Here's how the part is built. I have some questions about the finished solid (model axes, mm). Face numbers are marked on the shaded views. A direction names the side the tool comes from. Coordinates: 2 decimals unless noted, no trailing zeros. Write each loop counter-clockwise with the first axis right and the second up, starting at its lowest first coordinate (ties: lowest second). Pieces come first, ordered by that corner, then holes.
(1) Please list where these lines run through material, in increasing order: probe 1 along Y at (x, z) = (36, 48); probe 2 along X at (y, z) = (23, 12); probe 3 along Z at (x, y) = (24, 10).
(2) Imagine slicing it at A-A, the plane z = 24.5. List the corners of the cut face in (x, y) for me.
(3) Thinking about a two-plate mould opening in Z: for the marked faces 1, 2 and 3, which applies, released by +Z, released by -Z, zero draft, split by the parting line, or undercut?
(4) Imagine slicing it at D-D, the plane z = 30.5. List the corners of the cut face in (x, y) for me.
(5) Which directions (+Z, -Z, +X, -X, +Y, -Y) give clear straight access to the entire face, cutting with the end or side of a thin tool? Please do the marked faces 4, 5 and 6.
(6) Imagine slicing it at B-B, the plane x = 18. List the corners of the cut face in (y, z) for me.
(7) Imagine slicing it at C-C, the plane y = 8.5. List the corners of the cut face in (x, z) for me, plus the area to 3 significant figures.
(8) For pin 1 Ø1 at (x, y) = (9, 15) entering from +Z; pin 2 Ø7.5 at (x, y) = (-6.5, 8.5) entering from -Z; pin 3 Ø4 at (y, z) = (18, 3.5) entering from +X, each with a flat end and sliding along its axis, tell me the tip position at first contact or that it passes through.
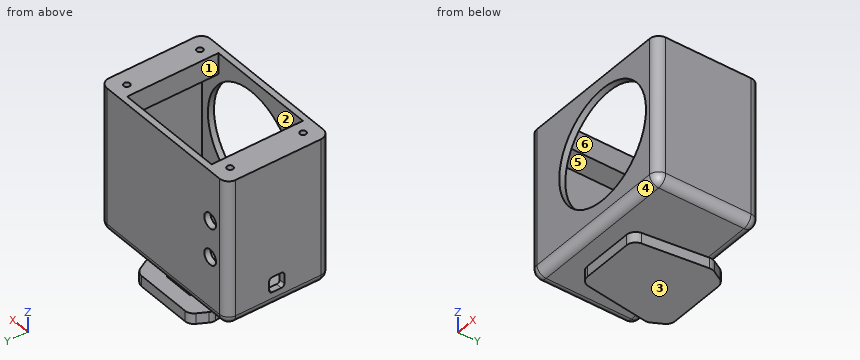
```python
from build123d import *

# Parameters (mm, degrees)
BOSS_EXTRUDE1_DEPTH  = 3.5
SKETCH2_W            = 10
SKETCH2_H            = 3
BOSS_EXTRUDE2_DEPTH  = 5
SKETCH3_W            = 50
SKETCH3_H            = 24
BOSS_EXTRUDE3_DEPTH  = 3
SKETCH4_W            = 50
SKETCH4_H            = 3
BOSS_EXTRUDE4_DEPTH  = 35
SKETCH5_W            = 4
SKETCH5_H            = 29
CUT_EXTRUDE3_DEPTH   = 35
FILLET1_R            = 2
SKETCH6_R            = 3.175
BOSS_EXTRUDE6_DEPTH  = 35
FILLET2_R            = 3
SKETCH8_W            = 10
SKETCH8_H            = 5
BOSS_EXTRUDE7_DEPTH  = 10
SKETCH9_W            = 10
SKETCH9_H            = 5
BOSS_EXTRUDE8_DEPTH  = 10
SKETCH10_W           = 53.514300768
SKETCH10_H           = 42.489179877
CUT_EXTRUDE4_DEPTH   = 20
BOSS_EXTRUDE9_DEPTH  = 40
SKETCH13_W           = 40
SKETCH13_H           = 10
BOSS_EXTRUDE10_DEPTH = 20
SKETCH14_W           = 4
SKETCH14_H           = 20
CUT_EXTRUDE7_DEPTH   = 20
FILLET3_R            = 2
SKETCH16_W           = 40
SKETCH16_H           = 10
CUT_EXTRUDE9_DEPTH   = 4
SKETCH19_W           = 40
SKETCH19_H           = 10
CUT_EXTRUDE10_DEPTH  = 24
SKETCH20_W           = 4
SKETCH20_H           = 2
CUT_EXTRUDE11_DEPTH  = 44
FILLET4_R            = 10
SKETCH21_W           = 58
SKETCH21_H           = 24
BOSS_EXTRUDE11_DEPTH = 2
SKETCH22_W           = 54.310686521
SKETCH22_H           = 40
CUT_EXTRUDE14_DEPTH  = 57
SKETCH24_W           = 10
SKETCH24_H           = 5
CUT_EXTRUDE15_DEPTH  = 5
SKETCH25_W           = 52
SKETCH25_H           = 2
BOSS_EXTRUDE12_DEPTH = 45
SKETCH26_W           = 2
SKETCH26_H           = 45
BOSS_EXTRUDE13_DEPTH = 22
SKETCH27_R           = 2.5
CUT_EXTRUDE16_DEPTH  = 45
SKETCH29_W           = 2
SKETCH29_H           = 45
BOSS_EXTRUDE14_DEPTH = 10
SKETCH30_W           = 45
SKETCH30_H           = 2
BOSS_EXTRUDE15_DEPTH = 50
SKETCH31_R           = 18.5
CUT_EXTRUDE17_DEPTH  = 60
SKETCH32_W           = 3
SKETCH32_H           = 34
BOSS_EXTRUDE17_DEPTH = 2
SKETCH33_W           = 2
SKETCH33_H           = 34
BOSS_EXTRUDE18_DEPTH = 45
BOSS_EXTRUDE20_REACH = 76.256
SKETCH37_W           = 7
SKETCH37_H           = 7
SKETCH38_R           = 1
CUT_EXTRUDE18_DEPTH  = 16
FILLET5_R            = 3
FILLET6_R            = 3
SKETCH39_W           = 5
SKETCH39_H           = 5
CUT_EXTRUDE22_DEPTH  = 10
FILLET7_R            = 1
SKETCH40_W           = 7
SKETCH40_H           = 30
BOSS_EXTRUDE21_DEPTH = 0.2


# Some blends are built 0.0001 mm under size
with BuildPart() as part:
    # Sketch1 → Boss-Extrude1 (new body)
    with BuildSketch(Plane.XY):
        Polygon((0, 24), (3, 0), (25, 0), (28, 24), (25, 29.5), (3, 29.5), align=None)
    extrude(amount=-BOSS_EXTRUDE1_DEPTH)

    # Sketch2 → Boss-Extrude2 (add)
    with BuildSketch(Plane.XY):
        with Locations((14, 18)):
            Rectangle(SKETCH2_W, SKETCH2_H)
    extrude(amount=BOSS_EXTRUDE2_DEPTH)

    # Sketch3 → Boss-Extrude3 (add)
    with BuildSketch(Plane.XY.offset(5)):
        with Locations((14, 17.5)):
            Rectangle(SKETCH3_W, SKETCH3_H)
    extrude(amount=BOSS_EXTRUDE3_DEPTH)

    # Sketch4 → Boss-Extrude4 (add)
    with BuildSketch(Plane.XY.offset(8)):
        with Locations((14, 28)):
            Rectangle(SKETCH4_W, SKETCH4_H)
    extrude(amount=BOSS_EXTRUDE4_DEPTH)

    # Sketch5 → Cut-Extrude3 (cut)
    with BuildSketch(Plane(origin=(0, 29.5, 0), x_dir=(1, 0, 0), z_dir=(0, 1, 0))):
        with Locations((-6, -25.5)):
            Rectangle(SKETCH5_W, SKETCH5_H)
    extrude(amount=-CUT_EXTRUDE3_DEPTH, mode=Mode.SUBTRACT)

    # Fillet1
    fillet1_edges = [part.edges().sort_by_distance(p)[0] for p in [
        (-8, 28, 40),
        (-4, 28, 40),
        (-4, 28, 11),
        (-8, 28, 11),
    ]]
    fillet(fillet1_edges, radius=FILLET1_R - 0.0001)  # a hair under: the kernel refuses the full size

    # Sketch6 → Boss-Extrude6 (add)
    with BuildSketch(Plane(origin=(39, 0, 0), x_dir=(0, 0, -1), z_dir=(1, 0, 0))):
        with BuildLine():
            Line((-29.274917218, 38.5), (-43, 29.5))
            Line((-43, 29.5), (-5, 29.5))
            Line((-5, 29.5), (-21.725082782, 38.5))
            ThreePointArc((-21.725082782, 38.5), (-25.5, 40), (-29.274917218, 38.5))
        make_face()
        with Locations((-25.5, 34.5)):
            Circle(SKETCH6_R, mode=Mode.SUBTRACT)
    extrude(amount=-BOSS_EXTRUDE6_DEPTH)

    # Fillet2
    fillet2_edges = [part.edges().sort_by_distance(p)[0] for p in [
        (25, 0, -1.75),
        (3, 0, -1.75),
        (0, 24, -1.75),
        (3, 29.5, -1.75),
        (25, 29.5, -1.75),
        (28, 24, -1.75),
    ]]
    fillet(fillet2_edges, radius=FILLET2_R)

    # Sketch8 → Boss-Extrude7 (add)
    with BuildSketch(Plane(origin=(0, 19.5, 0), x_dir=(1, 0, 0), z_dir=(0, 1, 0))):
        with Locations((14, -2.5)):
            Rectangle(SKETCH8_W, SKETCH8_H)
    extrude(amount=BOSS_EXTRUDE7_DEPTH)

    # Sketch9 → Boss-Extrude8 (add)
    with BuildSketch(Plane.XZ.offset(-16.5)):
        with Locations((14, 2.5)):
            Rectangle(SKETCH9_W, SKETCH9_H)
    extrude(amount=BOSS_EXTRUDE8_DEPTH)

    # Sketch10 → Cut-Extrude4 (cut)
    with BuildSketch(Plane(origin=(0, 29.5, 0), x_dir=(1, 0, 0), z_dir=(0, 1, 0))):
        with Locations((30.757150384, -26.244589939)):
            Rectangle(SKETCH10_W, SKETCH10_H)
    extrude(amount=CUT_EXTRUDE4_DEPTH, mode=Mode.SUBTRACT)

    # Sketch11 → Boss-Extrude9 (add)
    with BuildSketch(Plane(origin=(39, 0, 0), x_dir=(0, 0, -1), z_dir=(1, 0, 0))):
        with BuildLine():
            Line((-43, 39.5), (-43, 29.5))
            Line((-43, 29.5), (-24, 29.5))
            Line((-24, 29.5), (-24, 34.5))
            ThreePointArc((-24, 34.5), (-27.535533906, 35.964466094), (-29, 39.5))
            Line((-29, 39.5), (-43, 39.5))
        make_face()
        with BuildLine():
            Line((-24, 34.5), (-24, 29.5))
            Line((-24, 29.5), (-5, 29.5))
            Line((-5, 29.5), (-5, 39.5))
            Line((-5, 39.5), (-19, 39.5))
            ThreePointArc((-19, 39.5), (-20.464466094, 35.964466094), (-24, 34.5))
        make_face()
    extrude(amount=-BOSS_EXTRUDE9_DEPTH)

    # Sketch13 → Boss-Extrude10 (add)
    with BuildSketch(Plane.XY.offset(43)):
        with Locations((19, 34.5)):
            Rectangle(SKETCH13_W, SKETCH13_H)
        Polygon((-1, 29.5), (-11, 29.5), (-11, 26.5), (39, 26.5), (39, 29.5), align=None)
    extrude(amount=BOSS_EXTRUDE10_DEPTH)

    # Sketch14 → Cut-Extrude7 (cut)
    with BuildSketch(Plane(origin=(0, 29.5, 0), x_dir=(1, 0, 0), z_dir=(0, 1, 0))):
        with Locations((-6, -48)):
            Rectangle(SKETCH14_W, SKETCH14_H)
    extrude(amount=-CUT_EXTRUDE7_DEPTH, mode=Mode.SUBTRACT)

    # Fillet3
    fillet3_edges = [part.edges().sort_by_distance(p)[0] for p in [
        (-8, 28, 58),
        (-4, 28, 58),
    ]]
    fillet(fillet3_edges, radius=FILLET3_R - 0.0001)  # a hair under: the kernel refuses the full size

    # Sketch16 → Cut-Extrude9 (cut)
    with BuildSketch(Plane(origin=(0, 0, 5), x_dir=(-1, 0, 0), z_dir=(0, 0, -1))):
        with Locations((-19, 34.5)):
            Rectangle(SKETCH16_W, SKETCH16_H)
    extrude(amount=-CUT_EXTRUDE9_DEPTH, mode=Mode.SUBTRACT)

    # Sketch19 → Cut-Extrude10 (cut)
    with BuildSketch(Plane.XY.offset(63)):
        with Locations((19, 34.5)):
            Rectangle(SKETCH19_W, SKETCH19_H)
    extrude(amount=-CUT_EXTRUDE10_DEPTH, mode=Mode.SUBTRACT)

    # Sketch20 → Cut-Extrude11 (cut)
    with BuildSketch(Plane.XY.offset(39)):
        with Locations((6, 31.5)):
            Rectangle(SKETCH20_W, SKETCH20_H)
        with Locations((32, 31.5)):
            Rectangle(SKETCH20_W, SKETCH20_H)
    extrude(amount=-CUT_EXTRUDE11_DEPTH, mode=Mode.SUBTRACT)

    # Fillet4
    # the kernel refuses this fillet: 10 mm, written as the material it takes off along each edge
    with BuildSketch(Plane(origin=(-26, 39.5, 9), x_dir=(0, 0, 1), z_dir=(1, 0, 0)), Plane(origin=(-26, 39.5, 39), x_dir=(0, -1, 0), z_dir=(1, 0, 0))) as fillet4_piece_1:
        with BuildLine():
            CenterArc((FILLET4_R, FILLET4_R), FILLET4_R, 180, 90)
            Line((0, FILLET4_R), (0, 0))
            Line((0, 0), (FILLET4_R, 0))
        make_face()
    extrude(amount=90, mode=Mode.SUBTRACT)

    # Sketch21 → Boss-Extrude11 (add)
    with BuildSketch(Plane.ZY.offset(11)):
        with Locations((34, 17.5)):
            Rectangle(SKETCH21_W, SKETCH21_H)
    extrude(amount=BOSS_EXTRUDE11_DEPTH)

    # Sketch22 → Cut-Extrude14 (cut)
    with BuildSketch(Plane.XY.offset(65)):
        with Locations((13.590652361, 21.5)):
            Rectangle(SKETCH22_W, SKETCH22_H)
    extrude(amount=-CUT_EXTRUDE14_DEPTH, mode=Mode.SUBTRACT)

    # Sketch24 → Cut-Extrude15 (cut)
    with BuildSketch(Plane(origin=(0, 29.5, 0), x_dir=(1, 0, 0), z_dir=(0, 1, 0))):
        with Locations((14, -2.5)):
            Rectangle(SKETCH24_W, SKETCH24_H)
    extrude(amount=-CUT_EXTRUDE15_DEPTH, mode=Mode.SUBTRACT)

    # Sketch25 → Boss-Extrude12 (add)
    with BuildSketch(Plane.XY.offset(8)):
        with Locations((13, 28.5)):
            Rectangle(SKETCH25_W, SKETCH25_H)
    extrude(amount=BOSS_EXTRUDE12_DEPTH)

    # Sketch26 → Boss-Extrude13 (add)
    with BuildSketch(Plane.XZ.offset(-27.5)):
        with Locations((-12, 30.5)):
            Rectangle(SKETCH26_W, SKETCH26_H)
    extrude(amount=BOSS_EXTRUDE13_DEPTH)

    # Sketch27 → Cut-Extrude16 (cut)
    with BuildSketch(Plane.XZ.offset(-27.5)):
        with Locations(Location((-6, 36.5, 0), (0, 0, 270))):
            Circle(SKETCH27_R)
        with Locations(Location((-6, 24.5, 0), (0, 0, 270))):
            Circle(SKETCH27_R)
    extrude(amount=-CUT_EXTRUDE16_DEPTH, mode=Mode.SUBTRACT)

    # Sketch29 → Boss-Extrude14 (add)
    with BuildSketch(Plane.XZ.offset(-5.5)):
        with Locations((-12, 30.5)):
            Rectangle(SKETCH29_W, SKETCH29_H)
        Polygon((-11, 8), (-13, 8), (-13, 5), (39, 5), (39, 8), align=None)
    extrude(amount=BOSS_EXTRUDE14_DEPTH)

    # Sketch30 → Boss-Extrude15 (add)
    with BuildSketch(Plane(origin=(-11, 0, 0), x_dir=(0, 0, -1), z_dir=(1, 0, 0))):
        with Locations((-30.5, -3.5)):
            Rectangle(SKETCH30_W, SKETCH30_H)
    extrude(amount=BOSS_EXTRUDE15_DEPTH)

    # Sketch31 → Cut-Extrude17 (cut)
    with BuildSketch(Plane.XZ.offset(-27.5)):
        with Locations(Location((18, 30.5, 0), (0, 0, 90))):
            Circle(SKETCH31_R)
    extrude(amount=CUT_EXTRUDE17_DEPTH, mode=Mode.SUBTRACT)

    # Sketch32 → Boss-Extrude17 (add)
    with BuildSketch(Plane(origin=(39, 0, 0), x_dir=(0, 0, -1), z_dir=(1, 0, 0))):
        with Locations((-6.5, 12.5)):
            Rectangle(SKETCH32_W, SKETCH32_H)
    extrude(amount=BOSS_EXTRUDE17_DEPTH)

    # Sketch33 → Boss-Extrude18 (add)
    with BuildSketch(Plane.XY.offset(8)):
        with Locations((40, 12.5)):
            Rectangle(SKETCH33_W, SKETCH33_H)
    extrude(amount=BOSS_EXTRUDE18_DEPTH)

    # Sketch37 → Boss-Extrude20 (add, up to next)
    with BuildSketch(Plane(origin=(0, -2.5, 0), x_dir=(1, 0, 0), z_dir=(0, 1, 0)), mode=Mode.PRIVATE) as boss_extrude20_sk1:
        with Locations((-7.5, -49.5)):
            Rectangle(SKETCH37_W, SKETCH37_H)
    boss_extrude20_tool1 = extrude(boss_extrude20_sk1.sketch, amount=BOSS_EXTRUDE20_REACH, mode=Mode.PRIVATE) - part.part
    # Sketch37 → Boss-Extrude20 (add, up to next)
    with BuildSketch(Plane(origin=(0, -2.5, 0), x_dir=(1, 0, 0), z_dir=(0, 1, 0)), mode=Mode.PRIVATE) as boss_extrude20_sk2:
        with Locations((35.5, -49.5)):
            Rectangle(SKETCH37_W, SKETCH37_H)
    boss_extrude20_tool2 = extrude(boss_extrude20_sk2.sketch, amount=BOSS_EXTRUDE20_REACH, mode=Mode.PRIVATE) - part.part
    add(boss_extrude20_tool1.solids().sort_by_distance((-7.5, -2.5, 49.5))[0])
    add(boss_extrude20_tool2.solids().sort_by_distance((35.5, -2.5, 49.5))[0])

    # Sketch38 → Cut-Extrude18 (cut)
    with BuildSketch(Plane.XY.offset(53)):
        with Locations((-8, 24.5)):
            Circle(SKETCH38_R)
        with Locations((-8, 0.5)):
            Circle(SKETCH38_R)
        with Locations((36, 24.5)):
            Circle(SKETCH38_R)
        with Locations((36, 0.5)):
            Circle(SKETCH38_R)
    extrude(amount=-CUT_EXTRUDE18_DEPTH, mode=Mode.SUBTRACT)

    # Fillet5
    fillet5_edges = [part.edges().sort_by_distance(p)[0] for p in [
        (-13, 29.5, 29),
        (-13, -4.5, 29),
        (41, 29.5, 29),
        (41, -4.5, 29),
    ]]
    fillet(fillet5_edges, radius=FILLET5_R)

    # Fillet6
    fillet6_edges = [part.edges().sort_by_distance(p)[0] for p in [
        (14, -4.5, 5),
        (14, 29.5, 5),
        (41, 12.5, 5),
        (-13, 12.5, 5),
        (40.121320344, 28.621320344, 5),
        (40.121320344, -3.621320344, 5),
        (-12.121320344, 28.621320344, 5),
        (-12.121320344, -3.621320344, 5),
    ]]
    fillet(fillet6_edges, radius=FILLET6_R)

    # Sketch39 → Cut-Extrude22 (cut)
    with BuildSketch(Plane.ZY.offset(13)):
        with Locations((12.5, 13)):
            Rectangle(SKETCH39_W, SKETCH39_H)
    extrude(amount=-CUT_EXTRUDE22_DEPTH, mode=Mode.SUBTRACT)

    # Fillet7
    fillet7_edges = [part.edges().sort_by_distance(p)[0] for p in [
        (-12, 10.5, 10),
        (-12, 15.5, 10),
        (-12, 15.5, 15),
        (-12, 10.5, 15),
    ]]
    fillet(fillet7_edges, radius=FILLET7_R)

    # Sketch40 → Boss-Extrude21 (add)
    with BuildSketch(Plane.XY.offset(46)):
        with Locations((-7.5, 12.5)):
            Rectangle(SKETCH40_W, SKETCH40_H)
        with Locations((35.5, 12.5)):
            Rectangle(SKETCH40_W, SKETCH40_H)
    extrude(amount=BOSS_EXTRUDE21_DEPTH)


solid = part.part
```
Recorded:
1. probe 1: y = -4.5 to -0.5, 1.5 to 23.5, 25.5 to 29.5
1. probe 2: x = -13 to -11, 39 to 41
1. probe 3: z = -3.5 to 0, 5 to 8
2. outline: (-13, -1.5) arc R3 ccw to (-10, -4.5) - (0.5, -4.5) - (0.5, -2.5) - (-11, -2.5) - (-11, 27.5) - (-8.5, 27.5) - (-8.5, 29.5) - (-10, 29.5) arc R3 ccw to (-13, 26.5) - close; (-3.5, 27.5) - (39, 27.5) - (39, -2.5) - (35.5, -2.5) - (35.5, -4.5) - (38, -4.5) arc R3 ccw to (41, -1.5) - (41, 26.5) arc R3 ccw to (38, 29.5) - (-3.5, 29.5) - close
3. face 1: zero draft
3. face 2: undercut
3. face 3: released by -Z
4. outline: (-13, -1.5) arc R3 ccw to (-10, -4.5) - (-0.5, -4.5) - (-0.5, -2.5) - (-11, -2.5) - (-11, 27.5) - (39, 27.5) - (39, -2.5) - (36.5, -2.5) - (36.5, -4.5) - (38, -4.5) arc R3 ccw to (41, -1.5) - (41, 26.5) arc R3 ccw to (38, 29.5) - (-10, 29.5) arc R3 ccw to (-13, 26.5) - close
5. face 4: -Z, +X, -X, -Y
5. face 5: none
5. face 6: +Z
6. outline: (-4.5, 8) arc R3 ccw to (-1.5, 5) - (6.5, 5) - (6.5, 0) - (0, 0) - (0, -3.5) - (29.5, -3.5) - (29.5, 0) - (24.5, 0) - (24.5, 5) - (26.5, 5) arc R3 ccw to (29.5, 8) - (29.5, 53) - (27.5, 53) - (27.5, 8) - (-2.5, 8) - (-2.5, 12) - (-4.5, 12) - close; (-4.5, 49) - (-2.5, 49) - (-2.5, 53) - (-4.5, 53) - close
7. outline: (-13, 8) arc R3 ccw to (-10, 5) - (9, 5) - (9, 0) - (1.94, 0) - (1.94, -3.5) - (26.06, -3.5) - (26.06, 0) - (19, 0) - (19, 5) - (38, 5) arc R3 ccw to (41, 8) - (41, 53) - (32, 53) - (32, 46) - (39, 46) - (39, 8) - (-11, 8) - (-11, 46) - (-4, 46) - (-4, 53) - (-13, 53) - close
7. area: 571 mm2
8. pin 1: stops at z = 8
8. pin 2: stops at z = 5
8. pin 3: stops at x = 39.66
